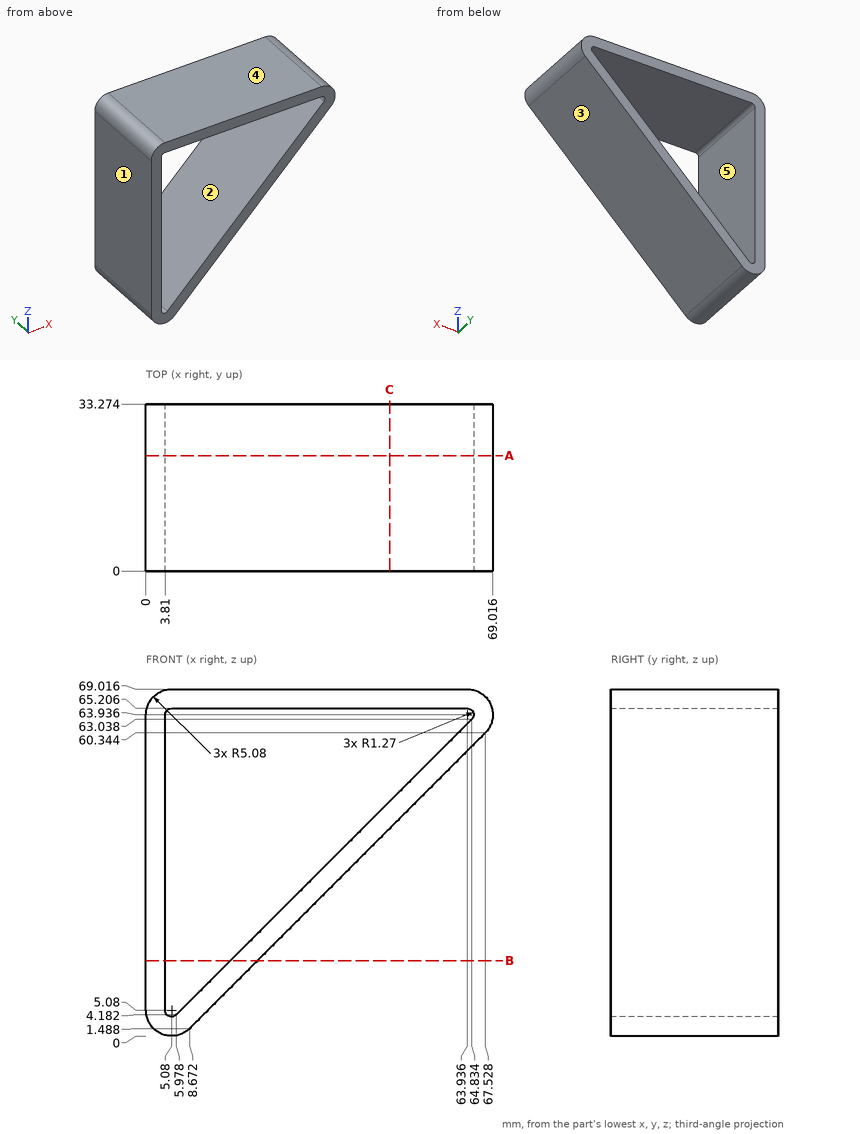
The drawing under review shows one solid part. Ordinate dimensions are in mm from its lowest x, y, z. A direction names the side the tool comes from. Coordinates: 2 decimals unless noted, no trailing zeros. Order: outer loops, then holes, each group sorted by start corner. A loop starts at its lowest first (then second) coordinate and runs counter-clockwise, first axis right, second up. Notation, with made-up numbers: (72.5, 29) -> (84.5, 29) arc R11 cw to (84.5, 37) -> close; hole circle Ø4 at (-23, 30). An arc over 180 degrees is marked (long way). Answer in a Markdown table with one row per item. Add a question column.
Item 1: Mouldability with a two-part tool opening along X and no side actions: class the marked faces 1, 2 and 3 as +X half, -X half, draft (parallel to the pull), parting line (faces both ways), or undercut.
Item 2: Machinability: for the marked faces 4 and 5, which of the approach directions +Z, -Z, +X, -X, +Y, -Y give a long, thin tool a straight path to every point of the face, cutting with its end or side? Answer none if there is none.
Item 3: We need section C-C on x = 48.5. Write out the cut boundary in (y, z), plus the area to 3 significant figures.
Item 4: Clearance check with flat-ended pins moving along their axes: pin 1 (1 mm diameter, centred on y = 21, z = 57, fed in from +X) (1 decimal); pin 2 (2 mm diameter, centred on x = 56, y = 15.5, fed in from -Z) (1 decimal); pin 3 (10 mm diameter, centred on x = 29.5, y = 15, fed in from -Z) (1 decimal). State where each tip first meets the part, or that it passes through.
Item 5: We need section B-B on z = 15. Write out the cut boundary in (x, y), plus the area to 3 significant figures.
Item 6: To check wall thickness, follow probe 1 along X at (y, z) = (27, 5.5) (1 decimal); probe 2 along Z at (x, y) = (13, 4) (1 decimal); probe 3 along X at (y, z) = (19.5, 42.5) (1 decimal). State the ranges of each line that lie inside material, in increasing order.
Item 7: We need section A-A on y = 23. Write out the cut boundary in (x, z).
Final values:
| question | item | result |
|---|---|---|
| 1 | face 1 | -X half |
| 1 | face 2 | undercut |
| 1 | face 3 | +X half |
| 2 | face 4 | +Z, +X, -X, +Y, -Y |
| 2 | face 5 | +Y, -Y |
| 3 | outline | (0, 41.32) -> (33.27, 41.32) -> (33.27, 46.7) -> (0, 46.7) -> close; (0, 65.21) -> (33.27, 65.21) -> (33.27, 69.02) -> (0, 69.02) -> close |
| 3 | area | 306 mm2 |
| 4 | pin 1 | stops at x = 64.7 |
| 4 | pin 2 | stops at z = 47.8 |
| 4 | pin 3 | stops at z = 17.3 |
| 5 | outline | (0, 0) -> (3.81, 0) -> (3.81, 33.27) -> (0, 33.27) -> close; (16.8, 0) -> (22.18, 0) -> (22.18, 33.27) -> (16.8, 33.27) -> close |
| 5 | area | 306 mm2 |
| 6 | probe 1 | x = 0 to 3.8, 7.3 to 12.7 |
| 6 | probe 2 | z = 5.8 to 11.2, 65.2 to 69 |
| 6 | probe 3 | x = 0 to 3.8, 44.3 to 49.7 |
| 7 | outline | (0, 5.08) arc R5.08 ccw to (8.67, 1.49) -> (67.53, 60.34) arc R5.08 ccw to (63.94, 69.02) -> (5.08, 69.02) arc R5.08 ccw to (0, 63.94) -> close; hole (3.81, 5.08) arc R1.27 ccw to (5.98, 4.18) -> (64.83, 63.04) arc R1.27 ccw to (63.94, 65.21) -> (5.08, 65.21) arc R1.27 ccw to (3.81, 63.94) -> close |
